Read the model definition and answer for the solid it produces. Units are mm, in the model's axes. Face numbers are marked on the shaded views. A direction names the side the tool comes from. Coordinates: 2 decimals unless noted, no trailing zeros. Write each loop counter-clockwise with the first axis right and the second up, starting at its lowest first coordinate (ties: lowest second). Pieces come first, ordered by that corner, then holes. Notation, with made-up numbers: (30.5, 81) -> (51.5, 81) arc R24 ccw to (51.5, 113) -> close; hole circle Ø2 at (38.25, 76). An arc over 180 degrees is marked (long way). Use CSV: the item, a comma, the result in double quotes.
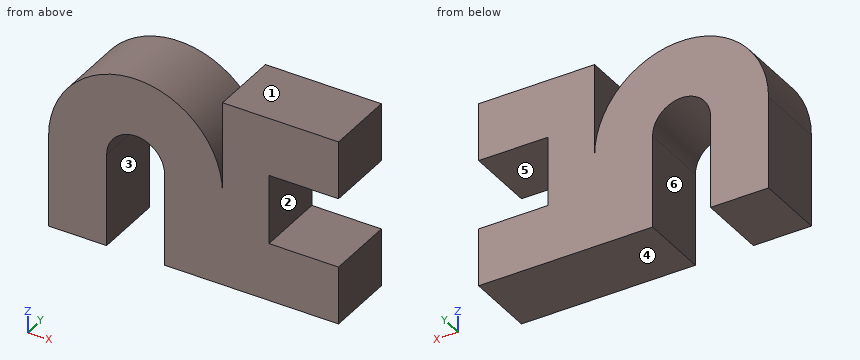
Autodesk Inventor part; units mm, degrees
ref_plane "YZ Plane" through (0, 0, 0) normal (1, 0, 0) x (0, 1, 0)
ref_plane "XZ Plane" through (0, 0, 0) normal (0, 1, 0) x (-1, 0, 0)
ref_plane "XY Plane" through (0, 0, 0) normal (0, 0, 1) x (1, 0, 0)
sketch "Sketch1" plane through (0, 0, 0) normal (0, 1, 0) x (-1, 0, 0)
  line L0 (0, 0) -> (0, -3)
  line L1 (0, -3) -> (-3, -3)
  line L2 (0, 0) -> (-3, 0)
  line L3 (-3, 0) -> (-3, 2.5)
  line L4 (-3, 2.5) -> (2, 2.5)
  line L5 (2, 2.5) -> (2, 0)
  line L6 (-3, -3) -> (-3, -5.5)
  line L7 (-3, -5.5) -> (4.5, -5.5)
  line L8 (4.5, -5.5) -> (4.5, -1.5)
  arc A0 (7, -1.5) -> (4.5, -1.5) centre (5.75, -1.5) ccw
  line L9 (7, -1.5) -> (7, -5.5)
  line L10 (7, -5.5) -> (9.5, -5.5)
  line L11 (9.5, -5.5) -> (9.5, -1.5)
  line L12 (2, 0) -> (2, -1.5)
  line L13 (4.5, -1.5) -> (2, -1.5) construction
  arc A1 (9.5, -1.5) -> (2, -1.5) centre (5.75, -1.5) ccw
  line L14 (2, -1.5) -> (2, -1.5)
  dimension "d0" = 3
  dimension "d1" = 3
  dimension "d2" = 2.5
  dimension "d3" = 5
  dimension "d4" = 2.5
  dimension "d5" = 7.5
  dimension "d6" = 2.5
  dimension "d7" = 1.25
  dimension "d8" = 2.5
  dimension "d9" = 2.5
  dimension "d10" = 3
  dimension "d13" = 0
  dimension "d14" = 2
extrude "Extrusion1" add sketch "Sketch1" along normal blind 3
equation "\"d2\" = d4"
equation "\"d8\" = d4"
equation "\"d10\" = d1"
properties part number "rubber_band_hook"
1. For a pull along X with two mould halves and no side action, classify the marked faces 1, 2 and 3 as pulls with the +X half, pulls with the -X half, needs draft (parallel to the pull), parting line crosses it, or undercut.
Solutions:
face 1,"needs draft"
face 2,"pulls with the +X half"
face 3,"undercut"
2. A cutting plane is placed at D-D (x = -5.75). Give the vertices of the cut face in (y, z).
Solutions:
outline,"(0, -0.25) -> (3, -0.25) -> (3, 2.25) -> (0, 2.25) -> close"
3. A cutting plane is placed at B-B (x = 0.25). Give the vertices of the cut face in (y, z).
Solutions:
outline,"(0, -5.5) -> (3, -5.5) -> (3, -3) -> (0, -3) -> close; (0, 0) -> (3, 0) -> (3, 2.5) -> (0, 2.5) -> close"
4. Find the intervals of material crossed by line 1 along X through (y, z) = (1.7, -2); line 2 along X through (y, z) = (0.2, -4); line 3 along Z through (x, y) = (1.75, 0.25), in increasing order.
Solutions:
line 1,"x = -9.5 to -7, -4.5 to 0"
line 2,"x = -9.5 to -7, -4.5 to 3"
line 3,"z = -5.5 to -3, 0 to 2.5"
5. A cutting plane is placed at A-A (z = -1.75). Give the vertices of the cut face in (x, y), and give its area (3 significant figures).
Solutions:
outline,"(-9.5, 0) -> (-7, 0) -> (-7, 3) -> (-9.5, 3) -> close; (-4.5, 0) -> (0, 0) -> (0, 3) -> (-4.5, 3) -> close"
area,"21.0 mm^2"
6. This flat-tipped pin is pushed along its axis until it touches: pin 1 Ø1.5 at (y, z) = (1.5, 0.5) entering from -X. Where does it stop, or does it pass through?
Solutions:
pin 1,"stops at x = -9.29"
7. A tool of negligible diameter and unlimited length cuts with its end or side. For the marked faces 4, 5 and 6, from which of +Z, -Z, +X, -X, +Y, -Y can it reach the whole face along a straight path? Write none if from no direction.
Solutions:
face 4,"-Z, +X, -X, +Y, -Y"
face 5,"+X, +Y, -Y"
face 6,"-Z, +Y, -Y"
8. A cutting plane is placed at C-C (y = 2.5). Give the vertices of the cut face in (x, z), and give its area (3 significant figures).
Solutions:
outline,"(-9.5, -5.5) -> (-7, -5.5) -> (-7, -1.5) arc R1.25 cw to (-4.5, -1.5) -> (-4.5, -5.5) -> (3, -5.5) -> (3, -3) -> (0, -3) -> (0, 0) -> (3, 0) -> (3, 2.5) -> (-2, 2.5) -> (-2, -1.5) arc R3.75 ccw to (-9.5, -1.5) -> close"
area,"70.6 mm^2"
